```python
from build123d import *

# Parameters (mm, degrees)
SKETCH1_R           = 2
BOSS_EXTRUDE1_DEPTH = 6.5
CHAMFER1_SIZE       = 0.5


with BuildPart() as part:
    # Sketch1 → Boss-Extrude1 (new body)
    with BuildSketch(Plane.XY):
        Circle(SKETCH1_R)
    extrude(amount=-BOSS_EXTRUDE1_DEPTH)

    # Chamfer1
    chamfer1_edges = [part.edges().sort_by_distance(p)[0] for p in [
        (-2, 0, 0),
    ]]
    chamfer(chamfer1_edges, length=CHAMFER1_SIZE)

    # Sketch2 → Revolve1 (revolve)
    with BuildSketch(Plane(origin=(0, 0, 0), x_dir=(0, 0, -1), z_dir=(1, 0, 0))):
        with BuildLine():
            Line((6.5, 0), (6.5, 3.5))
            ThreePointArc((6.5, 3.5), (8.485229955, 2.227844932), (9.257385023, 0))
            Line((9.257385023, 0), (6.5, 0))
        make_face()
    revolve(axis=Axis((0, 0, -3.742614977), (0, 0, -1)))


solid = part.part
```
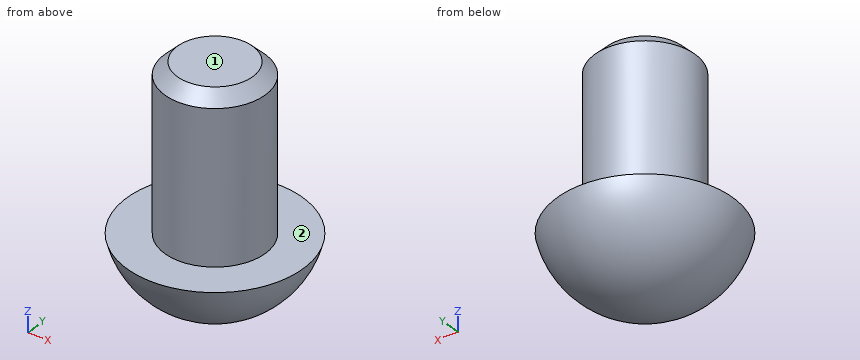
Read the model definition and answer for the solid it produces. Units are mm, in the model's axes. Face numbers are marked on the shaded views. A direction names the side the tool comes from. Coordinates: 2 decimals unless noted, no trailing zeros. Write each loop counter-clockwise with the first axis right and the second up, starting at its lowest first coordinate (ties: lowest second). Pieces come first, ordered by that corner, then holes. Notation, with made-up numbers: (22.25, 9.5) - (34.25, 9.5) arc R15 cw to (34.25, 21.5) - close; hole circle Ø6 at (33, 84.5). An arc over 180 degrees is marked (long way). Answer as a JSON object with one key per item and string values. Group by question number.
1. A cutting plane is placed at D-D (x = -2.25). Determine the outline of the cut face in (y, z).
2. A cutting plane is placed at C-C (z = -2). Determine the outline of the cut face in (x, y).
3. Which of the six approach directions +Z, -Z, +X, -X, +Y, -Y give full straight-line access (tool end or side, diameter ignored) to the marked faces 1 and 2?
4. Consider L1, parallel to Z at x = 2.25, y = -2.5; L2, parallel to Z at x = -1, y = 0; L3, parallel to Y at x = -1.25, z = -3.5. Determine where each line is inside the solid, lowest interval first. Write a range as [from, to].
5. Each of these flat-tipped pins is pushed along its axis until it touches: P1, Ø2, axis at y = 1, z = -6, coming from the +X side; P2, Ø3, axis at x = -2, z = -7.5, coming from the -Y side; P3, Ø1.5, axis at x = 1, y = 0, coming from the -Z side. Where does it stop, or does it pass through?
6. A cutting plane is placed at A-A (x = 0). Determine the outline of the cut face in (y, z).
Worked out:
{
 "1": {"outline": "(-2.68, -6.5) arc R2.81 ccw to (2.68, -6.5) - close"},
 "2": {"outline": "circle Ø4 at (0, 0)"},
 "3": {"face 1": "+Z, +X, -X, +Y, -Y", "face 2": "+Z"},
 "4": {"L1": "z = [-6.94, -6.5]", "L2": "z = [-9.12, 0]", "L3": "y = [-1.56, 1.56]"},
 "5": {"P1": "stops at x = 3.5", "P2": "stops at y = -3.39", "P3": "stops at z = -9.25"},
 "6": {"outline": "(-3.5, -6.5) arc R3.6 ccw to (3.5, -6.5) - (2, -6.5) - (2, -0.5) - (1.5, 0) - (-1.5, 0) - (-2, -0.5) - (-2, -6.5) - close"}
}
